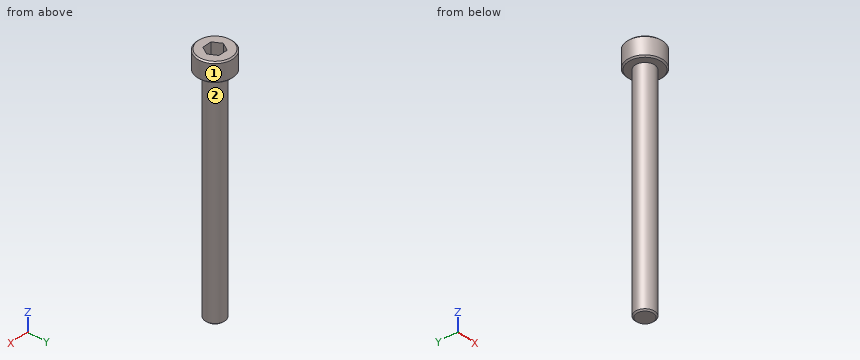
```python
from build123d import *

# Parameters (mm, degrees)
SKETCH_R     = 2.75
PAD_DEPTH    = 3
SKETCH001_R  = 1.5
PAD001_DEPTH = 35
POCKET_DEPTH = 4
CHAMFER_SIZE = 0.2


with BuildPart() as part:
    # Sketch → Pad (new body)
    with BuildSketch(Plane.XY):
        Circle(SKETCH_R)
    extrude(amount=PAD_DEPTH)

    # Sketch001 (on Face2 of Pad) → Pad001 (join)
    with BuildSketch(Plane(origin=(0, 0, 0), x_dir=(1, 0, 0), z_dir=(0, 0, -1))):
        Circle(SKETCH001_R)
    extrude(amount=PAD001_DEPTH)

    # Sketch002 (on DatumPlane) → Pocket (cut)
    with BuildSketch(Plane.XY.offset(3)):
        Polygon((0.721688, -1.25), (1.443376, 0), (0.721688, 1.25), (-0.721688, 1.25), (-1.443376, 0), (-0.721688, -1.25), align=None)
    extrude(amount=-POCKET_DEPTH, mode=Mode.SUBTRACT)

    # Chamfer
    chamfer_edges = [part.edges().sort_by_distance(p)[0] for p in [
        (-1.5, 0, -35),
        (-2.75, 0, 0),
        (-2.75, 0, 3),
    ]]
    chamfer(chamfer_edges, length=CHAMFER_SIZE)


solid = part.part
```
Input: part model. Units: mm. Frame: model coordinates. Face numbers are marked on the shaded views. A direction names the side the tool comes from. Coordinates: 2 decimals unless noted, no trailing zeros. Order: outer loops, then holes, each group sorted by start corner. A loop starts at its lowest first (then second) coordinate and runs counter-clockwise, first axis right, second up. Notation, with made-up numbers: (29, 74.5) - (41, 74.5) arc R19 cw to (41, 108.5) - close; hole circle Ø7 at (-24.5, -31.75). An arc over 180 degrees is marked (long way). Put each result on its own line as item: value.
1. Cut plane B-B on z = -1.5. Return the cut outline in (x, y), then the cut area to 3 significant figures.
Report:
outline: circle Ø3 at (0, 0)
area: 7.07 mm2
2. Cut plane A-A on x = 0. Return the cut outline in (y, z), then the cut area to 3 significant figures.
Report:
outline: (-2.75, 0.2) - (-2.55, 0) - (-1.5, 0) - (-1.5, -34.8) - (-1.3, -35) - (1.3, -35) - (1.5, -34.8) - (1.5, 0) - (2.55, 0) - (2.75, 0.2) - (2.75, 2.8) - (2.55, 3) - (1.25, 3) - (1.25, -1) - (-1.25, -1) - (-1.25, 3) - (-2.55, 3) - (-2.75, 2.8) - close
area: 111 mm2
3. Line query: line 1 along Z through (x, y) = (1.05, 0.3); line 2 along Z through (x, y) = (-1.85, 0.25); line 3 along Y through (x, z) = (0.05, -19.5). Output: solid intervals per line, ascending.
Report:
line 1: z = -35 to -1
line 2: z = 0 to 3
line 3: y = -1.5 to 1.5
4. Reachability of the marked faces 1 and 2 from +Z, -Z, +X, -X, +Y, -Y: full face, straight path, thin tool, end or side. Return the list, or none.
Report:
face 1: +Z, -Z
face 2: -Z
5. Contact query for flat-ended pins moving along their axis: pin 1 Ø1.5 at (y, z) = (0.5, -23) entering from +X; pin 2 Ø2 at (x, y) = (-0.5, 0) entering from +Z; pin 3 Ø1.5 at (y, z) = (1.5, -27.5) entering from -X. Output: stop coordinate, or through.
Report:
pin 1: stops at x = 1.5
pin 2: stops at z = 3
pin 3: stops at x = -1.3
